```python
from build123d import *

# Parameters (mm, degrees)
EXTRUDE_1_DEPTH     = 7
FILLET_1_R          = 10
CHAMFER_1_SIZE      = 5
SKETCH_3_W          = 3.25461804
SKETCH_3_H          = 54.107720412
CUT_EXTRUDE_2_DEPTH = 47.067962478
SKETCH_4_R          = 4
CUT_EXTRUDE_3_DEPTH = 47.067962478
SKETCH_5_W          = 10.028686974
SKETCH_5_H          = 29.771176491
EXTRUDE_2_DEPTH     = 19
CHAMFER_3_SIZE      = 19
CHAMFER_4_SIZE      = 3
SKETCH_6_R          = 2.514235327
CUT_EXTRUDE_4_DEPTH = 64.298215394
CHAMFER_5_SIZE      = 2


with BuildPart() as part:
    # Эскиз1 → Вытянуть1 (new body)
    with BuildSketch(Plane(origin=(0, 0, 0), x_dir=(0, 0, -1), z_dir=(1, 0, 0))):
        Polygon((-2.568460462, -29.775860751), (-8.159933039, -20.242473248), (-34.447863263, -20.242473248), (-34.447863263, 0), (27.095667874, 0), (27.095667874, -29.775860751), align=None)
    extrude(amount=-EXTRUDE_1_DEPTH)

    # Скругление1
    fillet_1_edges = [part.edges().sort_by_distance(p)[0] for p in [
        (-3.5, -20.242473248, 8.159933039),
    ]]
    fillet(fillet_1_edges, radius=FILLET_1_R)

    # Фаска1
    chamfer_1_edges = [part.edges().sort_by_distance(p)[0] for p in [
        (-3.5, -20.242473248, 34.447863263),
        (-3.5, 0, 34.447863263),
    ]]
    chamfer(chamfer_1_edges, length=CHAMFER_1_SIZE)

    # Эскиз3 → Вырез-Вытянуть2 (cut, through all)
    with BuildSketch(Plane(origin=(0, 0, 0), x_dir=(1, 0, 0), z_dir=(0, 1, 0))):
        with Locations((-7.6877425, -29.069741347)):
            Rectangle(SKETCH_3_W, SKETCH_3_H)
    extrude(amount=-CUT_EXTRUDE_2_DEPTH, mode=Mode.SUBTRACT)

    # Эскиз4 → Вырез-Вытянуть3 (cut, through all)
    with BuildSketch(Plane(origin=(0, 0, 0), x_dir=(0, 0, -1), z_dir=(1, 0, 0))):
        with Locations((-20.668500614, -11.046677749)):
            Circle(SKETCH_4_R)
    extrude(amount=-CUT_EXTRUDE_3_DEPTH, mode=Mode.SUBTRACT)

    # Эскиз5 → Вытянуть2 (add)
    with BuildSketch(Plane(origin=(0, 0, 0), x_dir=(0, 0, -1), z_dir=(1, 0, 0))):
        with Locations((13.06456917, -14.885588246)):
            Rectangle(SKETCH_5_W, SKETCH_5_H)
    extrude(amount=EXTRUDE_2_DEPTH)

    # Фаска3
    chamfer_3_edges = [part.edges().sort_by_distance(p)[0] for p in [
        (19, -29.771176491, -13.06456917),
    ]]
    chamfer(chamfer_3_edges, length=CHAMFER_3_SIZE - 0.0001)  # a hair under: the kernel refuses the full size

    # Фаска4
    chamfer_4_edges = [part.edges().sort_by_distance(p)[0] for p in [
        (19, 0, -13.06456917),
    ]]
    chamfer(chamfer_4_edges, length=CHAMFER_4_SIZE)

    # Эскиз6 → Вырез-Вытянуть4 (cut, through all)
    with BuildSketch(Plane(origin=(0, 0, -18.078912657), x_dir=(-1, 0, 0), z_dir=(0, 0, -1))):
        with Locations((-11.229341263, -8.118042122)):
            Circle(SKETCH_6_R)
    extrude(amount=-CUT_EXTRUDE_4_DEPTH, mode=Mode.SUBTRACT)

    # Фаска5
    chamfer_5_edges = [part.edges().sort_by_distance(p)[0] for p in [
        (0, -14.887930375, -27.095667874),
    ]]
    chamfer(chamfer_5_edges, length=CHAMFER_5_SIZE)


solid = part.part
```
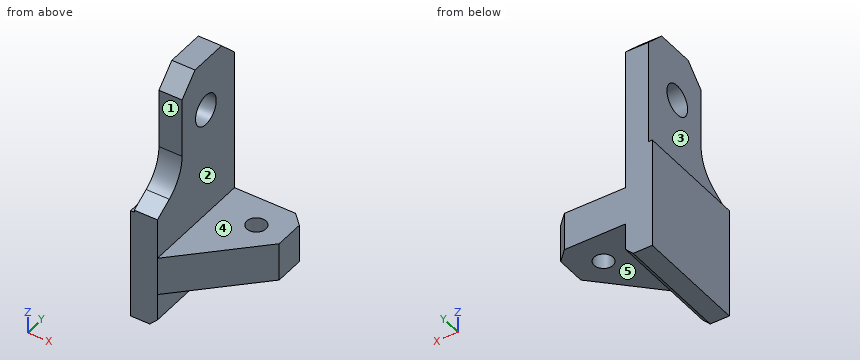
For this review, take the finished solid that the model builds, in its own axes (mm). Face numbers are marked on the shaded views. A direction names the side the tool comes from. Round coordinates to 2 decimals unless told otherwise and drop trailing zeros. Loops run counter-clockwise (first coordinate to the right, second up) from the corner with the lowest first, then second, coordinate; pieces in that order, holes last.
(1) Tool access review of the marked faces 1, 2, 3, 4 and 5: name each direction out of +Z, -Z, +X, -X, +Y, -Y from which nothing blocks a thin tool from reaching the whole face with its end or side.
Returned:
face 1: +Z, +X, -X, -Y
face 2: +X, +Y, -Y
face 3: +Z, -X, +Y, -Y
face 4: +Z, +X, +Y, -Y
face 5: -Z, +X, +Y, -Y
(2) We need section B-B (x = 11.5). Give the boundary of the cut face in (y, z).
Returned:
outline: (-18.27, -18.08) - (-10.62, -18.08) - (-10.62, -8.05) - (-18.27, -8.05) - close; (-5.62, -18.08) - (0, -18.08) - (0, -8.05) - (-5.62, -8.05) - close
(3) We need section C-C (y = -9.5). Give the boundary of the cut face in (x, z), plus the area to 3 significant figures.
Returned:
outline: (-7, -27.1) - (-2, -27.1) - (0, -25.1) - (0, -18.08) - (9.13, -18.08) - (9.13, -8.05) - (0, -8.05) - (0, 16.98) - (-6.06, 16.98) - (-6.06, 2.02) - (-7, 2.02) - close; (-6.06, 24.36) - (0, 24.36) - (0, 34.45) - (-6.06, 34.45) - close; (13.33, -18.08) - (19, -18.08) - (19, -8.05) - (13.33, -8.05) - close
area: 502 mm2
(4) Wall thickness on line 1 along Z through (x, y) = (4, -9.25); line 2 along X through (y, z) = (-8, -8); line 3 along X through (y, z) = (-15.75, 7): over which ranges is each line inside the solid? List them lowest first.
Returned:
line 1: z = -18.08 to -8.05
line 2: x = -7 to 0
line 3: x = -6.06 to 0
(5) We need section A-A (z = 18). Give the boundary of the cut face in (x, y).
Returned:
outline: (-6.06, -20.24) - (0, -20.24) - (0, -14.03) - (-6.06, -14.03) - close; (-6.06, -8.07) - (0, -8.07) - (0, 0) - (-6.06, 0) - close
(6) Clearance check with flat-ended pins moving along their axes: P1, Ø10.5, axis at y = -11.05, z = 20.67, coming from the -X side; P2, Ø1.5, axis at x = 3.5, y = -9.5, coming from the +Z side; P3, Ø9, axis at y = -20, z = 7.5, coming from the +X side. State where each tip first meets the part, or that it passes through.
Returned:
P1: stops at x = -6.06
P2: stops at z = -8.05
P3: stops at x = 0
(7) We need section D-D (x = -5). Give the boundary of the cut face in (y, z).
Returned:
outline: (-29.78, -27.1) - (0, -27.1) - (0, 29.45) - (-5, 34.45) - (-15.24, 34.45) - (-20.24, 29.45) - (-20.24, 13.89) arc R10 cw to (-25.18, 5.26) - (-29.78, 2.57) - close; hole circle Ø8 at (-11.05, 20.67)
